Autodesk Inventor part; units mm, degrees
ref_plane "YZ Plane" through (0, 0, 0) normal (1, 0, 0) x (0, 1, 0)
ref_plane "XZ Plane" through (0, 0, 0) normal (0, 1, 0) x (-1, 0, 0)
ref_plane "XY Plane" through (0, 0, 0) normal (0, 0, 1) x (1, 0, 0)
sketch "Sketch1" plane through (0, 0, 0) normal (0, 0, 1) x (1, 0, 0)
  line L0 (-10.4788, 3.5567) -> (22.1748, -35.3584)
  line L1 (-10.4788, 3.5567) -> (40.3212, 3.5567) construction
  line L2 (22.1748, -35.3584) -> (8.205, -87.4942)
  line L3 (8.205, -87.4942) -> (134.8162, -28.4545)
  line L4 (134.8162, -28.4545) -> (93.9992, 20.1894)
  line L5 (93.9992, 20.1894) -> (-10.4788, 3.5567)
  point P0 (0, 0)
  dimension "d0" = 50.8
  dimension "d1" = 50
  dimension "d2" = 53.975
  dimension "d3" = 125
  dimension "d4" = 139.7
  dimension "d5" = 50
  dimension "d6" = 63.5
  dimension "d7" = 75
extrude "Extrusion1" add sketch "Sketch1" along normal blind 3.175
sketch "Sketch2" plane through (0, 0, 3.175) normal (0, 0, 1) x (1, 0, 0)
  line L0 (-10.4788, 3.5567) -> (22.1748, -35.3584)
  line L1 (22.1748, -35.3584) -> (8.205, -87.4942)
  line L2 (22.1748, -35.3584) -> (9.9297, -20.7652)
  line L3 (22.1748, -35.3584) -> (17.2443, -53.7593)
  line L4 (9.9297, -20.7652) -> (3.7302, -22.1396)
  line L5 (17.2443, -53.7593) -> (11.0448, -55.1337)
  line L6 (15.9753, -36.7328) -> (3.7302, -22.1396)
  line L7 (15.9753, -36.7328) -> (11.0448, -55.1337)
  point P0 (0, 0)
  dimension "d10" = 19.05
  dimension "d11" = 19.05
  dimension "d12" = 6.35
  dimension "d13" = 6.35
  dimension "d14" = 6.35
extrude "Extrusion2" add sketch "Sketch2" against normal blind 3.175
sketch "Sketch3" plane through (0, 0, 0) normal (0, 0, -1) x (-1, 0, 0)
  line L0 (-17.2443, -53.7593) -> (-11.0448, -55.1337)
  line L1 (-11.0448, -55.1337) -> (-15.9753, -36.7328)
  line L2 (-15.9753, -36.7328) -> (-3.7302, -22.1396)
  line L3 (-3.7302, -22.1396) -> (-9.9297, -20.7652)
  line L4 (-3.7302, -22.1396) -> (-6.83, -21.4524)
  line L5 (-11.0448, -55.1337) -> (-14.1446, -54.4465)
  line L6 (-14.1446, -54.4465) -> (-19.0751, -36.0456)
  line L7 (-6.83, -21.4524) -> (-19.0751, -36.0456)
  point P0 (0, 0)
  dimension "d17" = 3.175
  dimension "d18" = 3.175
extrude "Extrusion3" add sketch "Sketch3" along normal blind 12.7
sketch "Sketch4" plane through (3.7302, -22.1396, -12.7) normal (-0.7660444, -0.6427876, 0) x (0, 0, 1)
  line L0 (0, -19.05) -> (0, 0)
  line L1 (15.875, -19.05) -> (0, -19.05)
  line L2 (0, -9.525) -> (6.35, -9.525)
  point P0 (12.7, 19.3577)
  dimension "d21" = 6.35
hole "Hole1" at (9.8528, -29.4362, -6.35) direction (0.7660444, 0.6427876, 0) diameter 6.35 end through all
sketch "Sketch5" plane through (15.9753, -36.7328, -12.7) normal (-0.9659258, 0.258819, 0) x (0, 0, 1)
  line L0 (0, -19.05) -> (0, 0)
  line L1 (15.875, -19.05) -> (0, -19.05)
  line L2 (0, -9.525) -> (6.35, -9.525)
  point P0 (12.7, 31.3464)
  dimension "d29" = 6.35
hole "Hole2" at (13.5101, -45.9332, -6.35) direction (0.9659258, -0.258819, 0) diameter 6.35 end through all
sketch "Sketch6" plane through (0, 0, 0) normal (0, 0, -1) x (-1, 0, 0)
  line L0 (-134.8162, -28.4545) -> (-93.9992, 20.1894)
  line L1 (-114.4077, -4.1326) -> (-103.5422, 8.8164)
  line L2 (-114.4077, -4.1326) -> (-125.2732, -17.0815)
  line L3 (-125.2732, -17.0815) -> (-130.1376, -12.9998)
  line L4 (-130.1376, -12.9998) -> (-108.4066, 12.8981)
  line L5 (-108.4066, 12.8981) -> (-103.5422, 8.8164)
  point P0 (0, 0)
  dimension "d37" = 16.9037
  dimension "d38" = 16.9037
  dimension "d39" = 6.35
  dimension "d40" = 33.8074
extrude "Extrusion4" add sketch "Sketch6" against normal blind 3.175
sketch "Sketch7" plane through (0, 0, 0) normal (0, 0, -1) x (-1, 0, 0)
  line L0 (-103.5422, 8.8164) -> (-108.4066, 12.8981)
  line L1 (-108.4066, 12.8981) -> (-130.1376, -12.9998)
  line L2 (-130.1376, -12.9998) -> (-125.2732, -17.0815)
  line L3 (-108.4066, 12.8981) -> (-130.1376, -12.9998)
  line L4 (-130.1376, -12.9998) -> (-127.7054, -15.0407)
  line L5 (-127.7054, -15.0407) -> (-105.9744, 10.8573)
  line L6 (-105.9744, 10.8573) -> (-108.4066, 12.8981)
  point P0 (0, 0)
  dimension "d43" = 3.175
extrude "Extrusion5" add sketch "Sketch7" along normal blind 12.7
sketch "Sketch8" plane through (108.4066, 12.8981, 3.175) normal (0.7660444, 0.6427876, 0) x (0, 0, -1)
  line L0 (15.875, 0) -> (15.875, -33.8074)
  line L1 (15.875, -16.9037) -> (9.525, -16.9037)
  point P0 (3.175, 59.8019)
  dimension "d46" = 6.35
hole "Hole3" at (119.2721, -0.0509, -6.35) direction (-0.7660444, -0.6427876, 0) diameter 6.35 end through all
properties part number "Right Bicep"
For this review, take the finished solid that the model builds, in its own axes (mm). A direction names the side the tool comes from. Coordinates: 2 decimals unless noted, no trailing zeros. Order: outer loops, then holes, each group sorted by start corner. A loop starts at its lowest first (then second) coordinate and runs counter-clockwise, first axis right, second up. Notation, with made-up numbers: (-23.75, 61) -> (9.25, 61) arc R26 ccw to (9.25, 86) -> close; hole circle Ø11 at (-17, -7). An arc over 180 degrees is marked (long way). Return JSON: item names as keys, results as strings.
1. We need section B-B on x = 44. Write out the cut boundary in (y, z) (3 decimals), and give its area (3 significant figures).
Answer block:
{"outline": "(-70.803, 0) -> (12.23, 0) -> (12.23, 3.175) -> (-70.803, 3.175) -> close", "area": "264 mm²"}
2. For line 1 (Z direction, x = 31, y = 5.5) (3 decimals); line 2 (Y direction, x = 6, z = 1); line 3 (Y direction, x = 121, z = -6.5), list the stretches that pass through material, from the lowest coordinate up. Write a range as from..to.
Answer block:
{"line 1": "0..3.175", "line 2": "-24.84..-21.64, -16.08..6.18", "line 3": "-7.05..-2.74"}
3. We need section D-D on y = -59. Write out the cut boundary in (x, z) (3 decimals).
Answer block:
{"outline": "(15.84, 0) -> (69.311, 0) -> (69.311, 3.175) -> (15.84, 3.175) -> close"}
4. Machinability: for faces 1 (the flat face through (128.28, -14.56, -2.89)), 2 (the flat face through (13.476, -46.062, -2.887)), 3 (the flat face through (98.84, 14.42, 1.57)), which of the approach directions +Z, -Z, +X, -X, +Y, -Y give a long, thin tool a straight path to every point of the face, cutting with its end or side? Answer none if there is none.
Answer block:
{"face 1": "+Z, -Z, +X", "face 2": "+Z, -Z, -X", "face 3": "+Z, -Z, +Y"}
5. We need section C-C on y = -38.5. Write out the cut boundary in (x, z) (3 decimals).
Answer block:
{"outline": "(15.502, -12.7) -> (18.417, -12.7) -> (18.417, 0) -> (113.274, 0) -> (113.274, 3.175) -> (15.502, 3.175) -> close"}
6. For pin 1 Ø4 at (y, z) = (-24.5, -5) entering from +X; pin 2 Ø5 at (x, y) = (27, -65) entering from -Z; pin 3 Ø1 at (x, z) = (36, 1.5) entering from +Y, all flat-tipped, find the tip position at first contact; note any pin that passes through.
Answer block:
{"pin 1": "x = 10.76", "pin 2": "z = 0", "pin 3": "y = 11.04"}
7. We need section A-A on z = -6.75. Write out the cut boundary in (x, y).
Answer block:
{"outline": "(3.73, -22.14) -> (7.83, -27.02) -> (9.99, -25.21) -> (6.83, -21.45) -> close; (11.04, -55.13) -> (14.14, -54.45) -> (15.42, -49.7) -> (12.69, -48.98) -> close; (11.88, -31.85) -> (15.98, -36.73) -> (14.33, -42.89) -> (17.05, -43.62) -> (19.08, -36.05) -> (14.03, -30.04) -> close; (105.97, 10.86) -> (114.82, 0.32) -> (117.25, 2.36) -> (108.41, 12.9) -> close; (118.86, -4.5) -> (127.71, -15.04) -> (130.14, -13) -> (121.3, -2.46) -> close"}
8. The part is to be moulded in two halves that separate along Y. For faces 4 (the flat face through (12.81, -54.742, -2.887)), 5 (the flat face through (119.12, 0.13, -2.89)), 6 (the flat face through (118, -1, -12.7)), 7 (the flat face through (-0.42, -8.43, 1.57)), say which applies: +Y half, -Y half, draft (parallel to the pull), parting line (faces both ways), or undercut.
Answer block:
{"face 4": "undercut", "face 5": "+Y half", "face 6": "draft", "face 7": "undercut"}
